```python
from build123d import *

# Parameters (mm, degrees)
SZKIC1_R                         = 6.5
DODANIE_WYCI_GNI_CIE1_DEPTH      = 6
SZKIC1_3_R                       = 6.5
SZKIC1_3_R_2                     = 3
DODANIE_WYCI_GNI_CIE2_DEPTH      = 16
DODANIE_WYCI_GNI_CIE3_DEPTH      = 16
DODANIE_WYCI_GNI_CIE3_DEPTH_BACK = 35
SZKIC1_4_R                       = 6.5
SZKIC1_4_R_2                     = 3
SFAZOWANIE1_SIZE                 = 2
SFAZOWANIE2_SIZE                 = 2


with BuildPart() as part:
    # Szkic1 → Dodanie-wyci_gni_cie1 (new body)
    with BuildSketch(Plane(origin=(0, 0, 0), x_dir=(1, 0, 0), z_dir=(0, 1, 0))):
        Polygon((5.484827557, 9.5), (-5.484827557, 9.5), (-10.969655115, 0), (-5.484827557, -9.5), (5.484827557, -9.5), (10.969655115, 0), align=None)
        with Locations(Location((0, 0, 0), (0, 0, 270))):
            Circle(SZKIC1_R, mode=Mode.SUBTRACT)
    extrude(amount=DODANIE_WYCI_GNI_CIE1_DEPTH)

    # Szkic1_3 → Dodanie-wyci_gni_cie2 (add)
    with BuildSketch(Plane(origin=(0, 0, 0), x_dir=(1, 0, 0), z_dir=(0, 1, 0))):
        with Locations(Location((0, 0, 0), (0, 0, 270))):
            Circle(SZKIC1_3_R)
        with Locations(Location((0, 0, 0), (0, 0, 270))):
            Circle(SZKIC1_3_R_2, mode=Mode.SUBTRACT)
    extrude(amount=DODANIE_WYCI_GNI_CIE2_DEPTH)

    # Szkic1_4 → Dodanie-wyci_gni_cie3 (add, two sides: drawn at the far end of the back side and taken through both)
    with BuildSketch(Plane(origin=(0, 0, 0), x_dir=(1, 0, 0), z_dir=(0, 1, 0)).offset(-DODANIE_WYCI_GNI_CIE3_DEPTH_BACK)):
        with Locations(Location((0, 0, 0), (0, 0, 270))):
            Circle(SZKIC1_4_R)
        with Locations(Location((0, 0, 0), (0, 0, 270))):
            Circle(SZKIC1_4_R_2, mode=Mode.SUBTRACT)
    extrude(amount=DODANIE_WYCI_GNI_CIE3_DEPTH + DODANIE_WYCI_GNI_CIE3_DEPTH_BACK)

    # Sfazowanie1
    sfazowanie1_edges = [part.edges().sort_by_distance(p)[0] for p in [
        (0, 16, -3),
    ]]
    chamfer(sfazowanie1_edges, length=SFAZOWANIE1_SIZE)

    # Sfazowanie2
    sfazowanie2_edges = [part.edges().sort_by_distance(p)[0] for p in [
        (0, -35, -3),
    ]]
    chamfer(sfazowanie2_edges, length=SFAZOWANIE2_SIZE)


solid = part.part
```
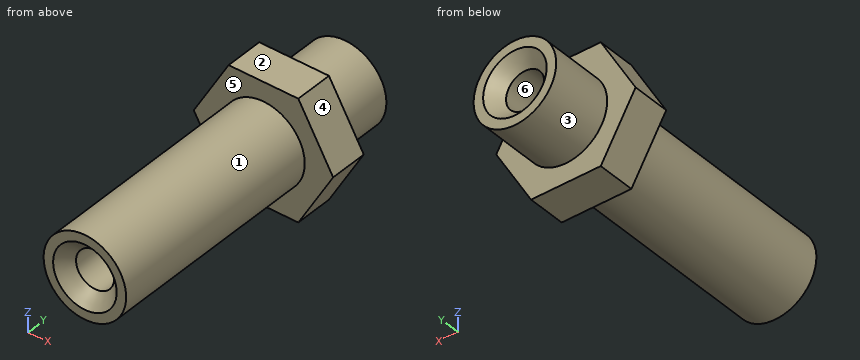
Could you check a few things on this model? Use its own coordinates, in mm. Face numbers are marked on the shaded views. A direction names the side the tool comes from. Coordinates: 2 decimals unless noted, no trailing zeros. Order: outer loops, then holes, each group sorted by start corner. A loop starts at its lowest first (then second) coordinate and runs counter-clockwise, first axis right, second up. Notation, with made-up numbers: M 3.25,6 L 35.25,6 A24 cw 35.25,19 Z; hole C -24.75,77.25 d10. An arc over 180 degrees is marked long. Use one line per item in the form item = value. Start each with the question number.
1. On a 3-axis mill with a long thin cutter (end or side, diameter ignored), from which of +Z, -Z, +X, -X, +Y, -Y can I reach the whole of each face in a straight line? I mean the marked faces 1, 2 and 3. Say none if no direction works.
2. Suppose I cut it at A-A on x = 0. Write out the boundary of the cut face in (y, z), then the cut area to 3 significant figures.
3. Suppose I cut it at B-B on y = -20. Write out the boundary of the cut face in (x, z), then the cut area to 3 significant figures.
4. Please list where these lines run through material, in increasing order: line 1 (X direction, y = 3, z = 0); line 2 (Z direction, x = -0.25, y = 7.5); line 3 (X direction, y = -19, z = 0).
5. We'd pull the mould along X, two halves only. Please class the marked faces 4, 5 and 6: +X half, -X half, draft (parallel to the pull), parting line (faces both ways), or undercut.
6. For pin 1 (4 mm diameter, centred on y = -26.5, z = -3.5, fed in from +X); pin 2 (2 mm diameter, centred on x = 2, y = -19.5, fed in from +Z); pin 3 (1 mm diameter, centred on y = 6, z = 5.5, fed in from +X), each with a flat end and sliding along its axis, tell me the tip position at first contact or that it passes through.
7. Suppose I cut it at C-C on x = 9.5. Write out the boundary of the cut face in (y, z).
Geometry says:
q1.face_1 = -Y
q1.face_2 = +Z, +X, -X, +Y, -Y
q1.face_3 = +Y
q2.outline = M -35,-6.5 L 0,-6.5 L 0,-9.5 L 6,-9.5 L 6,-6.5 L 16,-6.5 L 16,-5 L 14,-3 L -33,-3 L -35,-5 Z; M -35,5 L -33,3 L 14,3 L 16,5 L 16,6.5 L 6,6.5 L 6,9.5 L 0,9.5 L 0,6.5 L -35,6.5 Z
q2.area = 385 mm^2
q3.outline = C 0,0 d13; hole C 0,0 d6
q3.area = 104 mm^2
q4.line_1 = -10.97 to -3, 3 to 10.97
q4.line_2 = -6.5 to -2.99, 2.99 to 6.5
q4.line_3 = -6.5 to -3, 3 to 6.5
q5.face_4 = +X half
q5.face_5 = draft
q5.face_6 = undercut
q6.pin_1 = 6.32
q6.pin_2 = 6.42
q6.pin_3 = 8.08
q7.outline = M 0,-2.55 L 6,-2.55 L 6,2.55 L 0,2.55 Z
